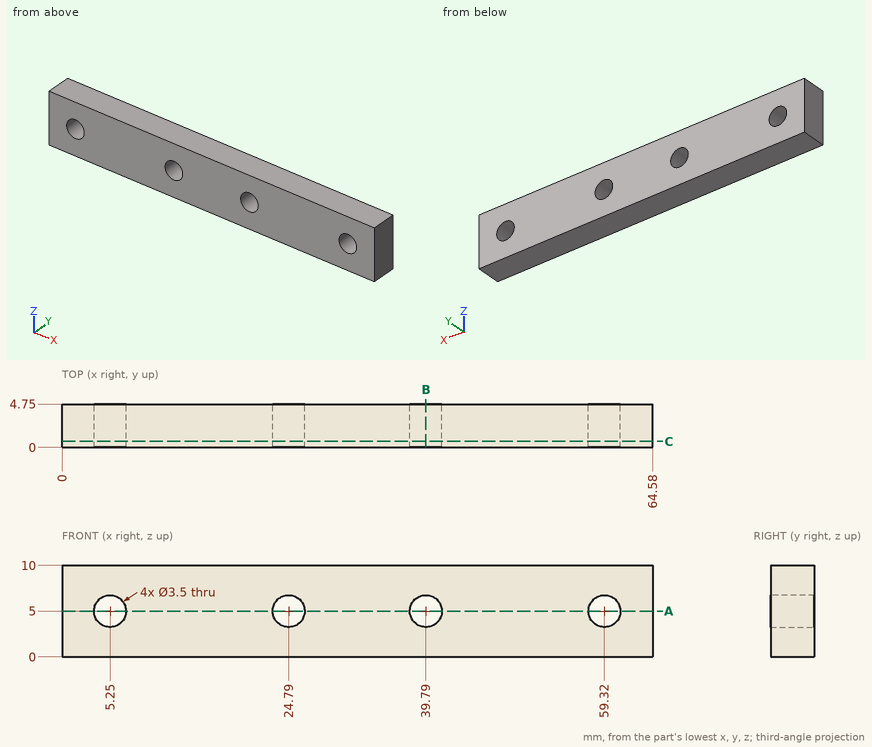
Print and shaded views of the part. All mm, measured from the part's lowest x, y and z. Give positions to 0.01 mm unless a question says otherwise; leave off trailing zeros. Loops run counter-clockwise (first coordinate to the right, second up) from the corner with the lowest first, then second, coordinate; pieces in that order, holes last. Notation, with made-up numbers: (-5.5, 6.25) -> (39.5, 6.25) arc R25 cw to (39.5, 31.25) -> close; hole circle Ø8 at (27, 47.25). An arc over 180 degrees is marked (long way). Use a Markdown table: item, result.
1. Wall check: L1, parallel to X at y = 1.6, z = 5; L2, parallel to X at y = 1.35, z = 4.75. Give the ranges that are in metal, low to high. Write a range as [from, to].
Check result:
| item | result |
|---|---|
| L1 | x = [0, 3.5], [7, 23.04], [26.54, 38.04], [41.54, 57.57], [61.07, 64.58] |
| L2 | x = [0, 3.52], [6.98, 23.06], [26.52, 38.06], [41.52, 57.59], [61.05, 64.58] |
2. Flat gauge pin, fed straight in: pin 1 (3 mm diameter, centred on x = 59.32, z = 5, fed in from -Y). Where does the tip first touch, or does it go through?
Check result:
| item | result |
|---|---|
| pin 1 | passes through |
3. Slice it at A-A (z = 5). List the corners of the cut face in (x, y).
Check result:
| item | result |
|---|---|
| outline | (0, 0) -> (3.5, 0) -> (3.5, 4.75) -> (0, 4.75) -> close; (7, 0) -> (23.04, 0) -> (23.04, 4.75) -> (7, 4.75) -> close; (26.54, 0) -> (38.04, 0) -> (38.04, 4.75) -> (26.54, 4.75) -> close; (41.54, 0) -> (57.57, 0) -> (57.57, 4.75) -> (41.54, 4.75) -> close; (61.07, 0) -> (64.58, 0) -> (64.58, 4.75) -> (61.07, 4.75) -> close |
4. Slice it at B-B (x = 39.79). List the corners of the cut face in (y, z).
Check result:
| item | result |
|---|---|
| outline | (0, 0) -> (4.75, 0) -> (4.75, 3.25) -> (0, 3.25) -> close; (0, 6.75) -> (4.75, 6.75) -> (4.75, 10) -> (0, 10) -> close |
5. Slice it at C-C (y = 0.65). List the corners of the cut face in (x, z).
Check result:
| item | result |
|---|---|
| outline | (0, 0) -> (64.58, 0) -> (64.58, 10) -> (0, 10) -> close; hole circle Ø3.5 at (5.25, 5); hole circle Ø3.5 at (24.79, 5); hole circle Ø3.5 at (39.79, 5); hole circle Ø3.5 at (59.32, 5) |
